Input: part model. Units: mm. Frame: model coordinates. A direction names the side the tool comes from. Give positions to 0.01 mm unless a question says otherwise; leave off trailing zeros. Loops run counter-clockwise (first coordinate to the right, second up) from the corner with the lowest first, then second, coordinate; pieces in that order, holes last. Notation, with made-up numbers: (-38.5, -39.5) - (-1.5, -39.5) arc R11 cw to (-1.5, -19.5) - close; hole circle Ø7 at (45.25, -23.75). An arc over 180 degrees is marked (long way). One line per item, written item: value.
from build123d import *

# Parameters (mm, degrees)
F1_DEPTH  = 100
F2_W      = 70
F2_H      = 15
F3_DEPTH  = 25.4
F4_W      = 25
F4_H      = 70
F5_DEPTH  = 50
F7_DEPTH  = 25
F8_R      = 10
F9_DEPTH  = 25.4
F10_R     = 7.5
F11_DEPTH = 25.4


with BuildPart() as f1:
    # F0 (on Front) → F1 (new body)
    with BuildSketch(Plane.XZ):
        Polygon((20, 45), (0, 45), (0, 0), (50, 0), (50, 10), (20, 10), align=None)
    extrude(amount=F1_DEPTH)

    # F2 (on face) → F3 (cut)
    with BuildSketch(Plane.YZ.offset(20)):
        with Locations((-49, 27.5)):
            Rectangle(F2_W, F2_H)
    extrude(amount=-F3_DEPTH, mode=Mode.SUBTRACT)

    # F4 (on Right) → F5 (join)
    with BuildSketch(Plane.YZ):
        with Locations((12.5, 35)):
            Rectangle(F4_W, F4_H)
    extrude(amount=F5_DEPTH)

    # F6 (on face) → F7 (join)
    with BuildSketch(Plane(origin=(0, 25, 0), x_dir=(-1, 0, 0), z_dir=(0, 1, 0))):
        with BuildLine():
            ThreePointArc((0, 70), (-25, 95), (-50, 70))
            Line((-50, 70), (0, 70))
        make_face()
    extrude(amount=-F7_DEPTH)

    # F8 (on face) → F9 (cut)
    with BuildSketch(Plane(origin=(0, 25, 0), x_dir=(-1, 0, 0), z_dir=(0, 1, 0))):
        with Locations((-25, 70)):
            Circle(F8_R)
    extrude(amount=-F9_DEPTH, mode=Mode.SUBTRACT)

    # F10 (on face) → F11 (cut)
    with BuildSketch(Plane.XY.offset(10)):
        with Locations((35, -25)):
            Circle(F10_R)
        with Locations((35, -75)):
            Circle(F10_R)
    extrude(amount=-F11_DEPTH, mode=Mode.SUBTRACT)


solid = f1.part
Item 1: Section C-C, the plane x = 25. Output: boundary loops of the cut face in (y, z).
Verdict:
outline: (-100, 0) - (25, 0) - (25, 60) - (0, 60) - (0, 10) - (-100, 10) - close; (0, 80) - (25, 80) - (25, 95) - (0, 95) - close
Item 2: Section D-D, the plane x = 10. Output: boundary loops of the cut face in (y, z).
Verdict:
outline: (-100, 0) - (25, 0) - (25, 90) - (0, 90) - (0, 45) - (-100, 45) - close; hole (-84, 20) - (-14, 20) - (-14, 35) - (-84, 35) - close
Item 3: Draft query along Y for faces 1 (the face through (25, -38, 0)), 2 (the face through (10, -49, 35)), 3 (the face through (14, -100, 18)), 4 (the face through (29.5, -19.9, 5.1)). Return one class per face: pulls with the +Y half, pulls with the -Y half, needs draft (parallel to the pull), parting line crosses it, or undercut.
Verdict:
face 1: needs draft
face 2: undercut
face 3: pulls with the -Y half
face 4: undercut
Item 4: Pin query (flat end, axial travel): P1, Ø10, axis at x = 7.5, y = -51, coming from the +Z side; P2, Ø8, axis at x = 29.5, y = -34, coming from the +Z side; P3, Ø18, axis at x = 25, z = 70, coming from the +Y side; P4, Ø8, axis at y = -13.5, z = 42, coming from the +X side. Return the tip coordinate at first contact, or that it passes through.
Verdict:
P1: stops at z = 45
P2: stops at z = 10
P3: passes through
P4: stops at x = 20
Item 5: Section B-B, the plane z = 32.5. Output: boundary loops of the cut face in (x, y), and give its area (3 significant figures).
Verdict:
outline: (0, -100) - (20, -100) - (20, -84) - (0, -84) - close; (0, -14) - (20, -14) - (20, 0) - (50, 0) - (50, 25) - (0, 25) - close
area: 1,850 mm^2
Item 6: Section A-A, the plane y = -19. Output: boundary loops of the cut face in (x, z), and give its area (3 significant figures).
Verdict:
outline: (0, 0) - (30.5, 0) - (30.5, 10) - (20, 10) - (20, 20) - (0, 20) - close; (0, 35) - (20, 35) - (20, 45) - (0, 45) - close; (39.5, 0) - (50, 0) - (50, 10) - (39.5, 10) - close
area: 810 mm^2
Item 7: Access query for faces 5 (the face through (35, -49, 10)), 6 (the face through (10, -49, 45)), 7 (the face through (10, -14, 27)), 8 (the face through (25, 25, 48)). Directions: +Z, -Z, +X, -X, +Y, -Y. A direction counts if a zero-diameter tool reaches every point of the face in a straight line with its end or side. Return the directions, or none.
Verdict:
face 5: +Z, +X, -Y
face 6: +Z, +X, -X, -Y
face 7: +X, -X
face 8: +Z, -Z, +X, -X, +Y
Item 8: Material intervals for L1, parallel to Y at x = 35, z = 5.5; L2, parallel to Z at x = 17, y = -76; L3, parallel to X at y = -5, z = 43, sorted ascending.
Verdict:
L1: y = -100 to -82.5, -67.5 to -32.5, -17.5 to 25
L2: z = 0 to 20, 35 to 45
L3: x = 0 to 20
